The model under review builds one solid part; all positions refer to its coordinate system, in mm. Face numbers are marked on the shaded views. A direction names the side the tool comes from. Coordinates: 2 decimals unless noted, no trailing zeros. Write each loop counter-clockwise with the first axis right and the second up, starting at its lowest first coordinate (ties: lowest second). Pieces come first, ordered by that corner, then holes. Notation, with made-up numbers: (-33.75, -29) - (-15.75, -29) arc R10 ccw to (-15.75, -13) - close; hole circle Ø4 at (-29, 64). An arc over 180 degrees is marked (long way). Put each result on its own line as item: value. Start each with the question number.
Item 1: To check wall thickness, follow L1, parallel to Y at x = 0, z = 5.25; L2, parallel to Z at x = 0.5, y = -3; L3, parallel to X at y = -4.25, z = 7.75. State the ranges of each line that lie inside material, in increasing order. Write a range as [from, to].
Item 2: Consider section D-D on z = 2.25. Give the boundary of the cut face in (x, y).
Item 3: For pin 1 (3 mm diameter, centred on x = 3, y = -1.5, fed in from -Z), flat-tipped, find the tip position at first contact; note if it passes through.
Item 4: Machinability: for the marked faces 1, 2 and 3, which of the approach directions +Z, -Z, +X, -X, +Y, -Y give a long, thin tool a straight path to every point of the face, cutting with its end or side? Answer none if there is none.
Item 5: Mouldability with a two-part tool opening along Y and no side actions: class the marked faces 4, 5 and 6 as pulls with the +Y half, pulls with the -Y half, needs draft (parallel to the pull), parting line crosses it, or undercut.
Item 6: Consider section B-B on x = -3.5. Give the boundary of the cut face in (y, z), then the cut area to 3 significant figures.
Item 7: Consider section C-C on y = -1.5. Give the boundary of the cut face in (x, z).
Item 8: Consider section A-A on x = 0. Give the boundary of the cut face in (y, z).
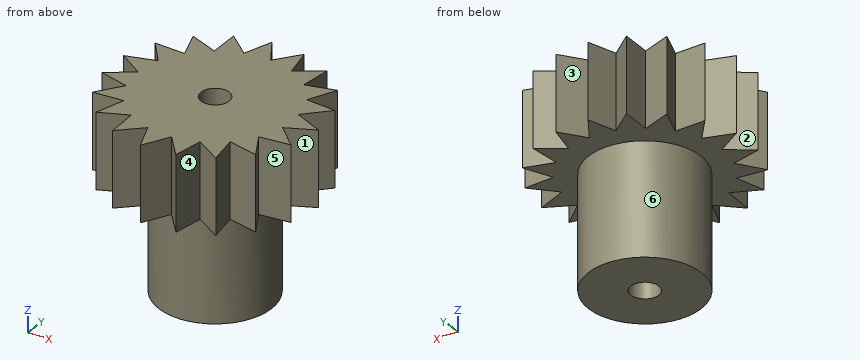
```python
from build123d import *

# Parameters (mm, degrees)
F0_R     = 3
F1_DEPTH = 6
F2_R     = 3
F3_DEPTH = 4
F4_R     = 0.75
F5_DEPTH = 25.4


with BuildPart() as f1:
    # F0 (on Top) → F1 (new body)
    with BuildSketch(Plane.XY):
        Circle(F0_R)
    extrude(amount=F1_DEPTH)

    # F2 (on face) → F3 (join)
    with BuildSketch(Plane.XY.offset(6)):
        Polygon((4.04302, -0.693343), (5.5, 0), (3.986969, 0.681121), (5.168309, 1.881111), (3.582234, 1.998583), (4.281007, 3.452967), (2.742315, 3.050646), (2.932624, 4.652925), (1.607039, 3.774144), (1.268387, 5.351747), (0.298678, 4.091152), (-0.53246, 5.474165), (-1.041851, 3.967528), (-2.275959, 5.006996), (-2.270169, 3.416587), (-3.774329, 4.000555), (-3.253981, 2.497667), (-4.86619, 2.563239), (-3.887328, 1.309739), (-5.433944, 0.849853), (-4.101995, -0.019253), (-5.416443, -0.955065), (-3.874862, -1.346171), (-4.81557, -2.657119), (-3.230392, -2.528102), (-3.696043, -4.072992), (-2.237997, -3.437747), (-2.178439, -5.050189), (-1.004562, -3.977133), (-0.426208, -5.483461), (0.337069, -4.088168), (1.371926, -5.326145), (1.642396, -3.758892), (3.022299, -4.595183), (2.770831, -3.024769), (4.34716, -3.369303), (3.600837, -1.964868), (5.203815, -1.780537), align=None)
        Circle(F2_R, mode=Mode.SUBTRACT)
        Circle(F2_R)
    extrude(amount=F3_DEPTH)

    # F4 (on face) → F5 (cut)
    with BuildSketch(Plane(origin=(0, 0, 0), x_dir=(1, 0, 0), z_dir=(0, 0, -1))):
        Circle(F4_R)
    extrude(amount=-F5_DEPTH, mode=Mode.SUBTRACT)


solid = f1.part
```
Report:
1. L1: [-3, -0.75], [0.75, 3]
1. L2: [6, 10]
1. L3: [-2.21, -1.3], [-0.9, 0.25], [0.47, 1.56], [2.45, 2.97]
2. outline: circle Ø6 at (0, 0); hole circle Ø1.5 at (0, 0)
3. pin 1: z = 0
4. face 1: +Z, -Z, +X
4. face 2: +Z, -Z, -X
4. face 3: +Z, -Z, +Y
5. face 4: pulls with the -Y half
5. face 5: undercut
5. face 6: parting line crosses it
6. outline: (-3.99, 6) - (-3.42, 6) - (-3.42, 10) - (-3.99, 10) - close; (-2.55, 6) - (2.51, 6) - (2.51, 10) - (-2.55, 10) - close; (3.21, 6) - (3.89, 6) - (3.89, 10) - (3.21, 10) - close
6. area: 25.2 mm²
7. outline: (-3.99, 6) - (-2.6, 6) - (-2.6, 0) - (2.6, 0) - (2.6, 6) - (4.9, 6) - (4.9, 10) - (-3.99, 10) - close
8. outline: (-4.7, 6) - (-3, 6) - (-3, 0) - (-0.75, 0) - (-0.75, 10) - (-4.7, 10) - close; (0.75, 0) - (3, 0) - (3, 6) - (4.59, 6) - (4.59, 10) - (0.75, 10) - close
